from build123d import *

# Parameters (mm, degrees)
SKETCH_25_W          = 70
SKETCH_25_H          = 30
SKETCH_25_R          = 1.5
EXTRUDE_9_DEPTH      = 4
SKETCH_26_W          = 6
SKETCH_26_H          = 6
SKETCH_26_R          = 1.5
EXTRUDE_10_DEPTH     = 4
FILLET_3_R           = 1
EXTRUDE_11_DEPTH     = 6
SKETCH_28_W          = 6
SKETCH_28_H          = 18
EXTRUDE_12_DEPTH     = 2
SKETCH_29_R          = 5
CUT_EXTRUDE_15_DEPTH = 3
FILLET_4_R           = 5


with BuildPart() as part:
    # 草图25 → 凸台-拉伸9 (new body)
    with BuildSketch(Plane(origin=(0, 0, 0), x_dir=(1, 0, 0), z_dir=(0, 1, 0))):
        Rectangle(SKETCH_25_W, SKETCH_25_H)
        with Locations(Location((-32, 12, 0), (0, 0, 270))):
            Circle(SKETCH_25_R, mode=Mode.SUBTRACT)
        with Locations(Location((32, 12, 0), (0, 0, 270))):
            Circle(SKETCH_25_R, mode=Mode.SUBTRACT)
        with Locations(Location((32, -12, 0), (0, 0, 270))):
            Circle(SKETCH_25_R, mode=Mode.SUBTRACT)
        with Locations(Location((-32, -12, 0), (0, 0, 270))):
            Circle(SKETCH_25_R, mode=Mode.SUBTRACT)
    extrude(amount=EXTRUDE_9_DEPTH)

    # 草图26 → 凸台-拉伸10 (add)
    # profile 1 of 4: a face of its own
    with BuildSketch(Plane(origin=(0, 4, 0), x_dir=(1, 0, 0), z_dir=(0, 1, 0))):
        with Locations((-32, 12)):
            Rectangle(SKETCH_26_W, SKETCH_26_H)
        with Locations(Location((-32, 12, 0), (0, 0, 270))):
            Circle(SKETCH_26_R, mode=Mode.SUBTRACT)
    # profile 2 of 4: a face of its own
    with BuildSketch(Plane(origin=(0, 4, 0), x_dir=(1, 0, 0), z_dir=(0, 1, 0))):
        with Locations((-32, -12)):
            Rectangle(SKETCH_26_W, SKETCH_26_H)
        with Locations(Location((-32, -12, 0), (0, 0, 270))):
            Circle(SKETCH_26_R, mode=Mode.SUBTRACT)
    # profile 3 of 4: a face of its own
    with BuildSketch(Plane(origin=(0, 4, 0), x_dir=(1, 0, 0), z_dir=(0, 1, 0))):
        with Locations((32, -12)):
            Rectangle(SKETCH_26_W, SKETCH_26_H)
        with Locations(Location((32, -12, 0), (0, 0, 270))):
            Circle(SKETCH_26_R, mode=Mode.SUBTRACT)
    # profile 4 of 4: a face of its own
    with BuildSketch(Plane(origin=(0, 4, 0), x_dir=(1, 0, 0), z_dir=(0, 1, 0))):
        with Locations((32, 12)):
            Rectangle(SKETCH_26_W, SKETCH_26_H)
        with Locations(Location((32, 12, 0), (0, 0, 270))):
            Circle(SKETCH_26_R, mode=Mode.SUBTRACT)
    extrude(amount=EXTRUDE_10_DEPTH)

    # 圆角3
    fillet_3_edges = [part.edges().sort_by_distance(p)[0] for p in [
        (-35, 4, -15),
        (35, 4, -15),
        (35, 4, 15),
        (-35, 4, 15),
    ]]
    fillet(fillet_3_edges, radius=FILLET_3_R)

    # 草图27 → 凸台-拉伸11 (add)
    with BuildSketch(Plane.XZ):
        with BuildLine():
            Line((-42.4, 0), (-35, 0))
            Line((-35, 0), (-35, 10))
            Line((-35, 10), (-55, 10))
            Line((-55, 10), (-55, 0))
            Line((-55, 0), (-47.6, 0))
            ThreePointArc((-47.6, 0), (-45, 2.6), (-42.4, 0))
        make_face()
        with BuildLine():
            Line((-35, -10), (-35, 0))
            Line((-35, 0), (-42.4, 0))
            ThreePointArc((-42.4, 0), (-45, -2.6), (-47.6, 0))
            Line((-47.6, 0), (-55, 0))
            Line((-55, 0), (-55, -10))
            Line((-55, -10), (-35, -10))
        make_face()
        with BuildLine():
            ThreePointArc((42.4, 0), (45, 2.6), (47.6, 0))
            Line((47.6, 0), (55, 0))
            Line((55, 0), (55, 10))
            Line((55, 10), (35, 10))
            Line((35, 10), (35, 0))
            Line((35, 0), (42.4, 0))
        make_face()
        with BuildLine():
            Line((55, 0), (47.6, 0))
            ThreePointArc((47.6, 0), (45, -2.6), (42.4, 0))
            Line((42.4, 0), (35, 0))
            Line((35, 0), (35, -10))
            Line((35, -10), (55, -10))
            Line((55, -10), (55, 0))
        make_face()
    extrude(amount=-EXTRUDE_11_DEPTH)

    # 草图28 → 凸台-拉伸12 (add)
    with BuildSketch(Plane(origin=(0, 4, 0), x_dir=(1, 0, 0), z_dir=(0, 1, 0))):
        with Locations((-32, 0)):
            Rectangle(SKETCH_28_W, SKETCH_28_H)
        with Locations((32, 0)):
            Rectangle(SKETCH_28_W, SKETCH_28_H)
    extrude(amount=EXTRUDE_12_DEPTH)

    # 草图29 → 切除-拉伸15 (cut)
    with BuildSketch(Plane(origin=(0, 6, 0), x_dir=(1, 0, 0), z_dir=(0, 1, 0))):
        with Locations(Location((-45, 0, 0), (0, 0, 270))):
            Circle(SKETCH_29_R)
        with Locations(Location((45, 0, 0), (0, 0, 270))):
            Circle(SKETCH_29_R)
    extrude(amount=-CUT_EXTRUDE_15_DEPTH, mode=Mode.SUBTRACT)

    # 圆角4
    fillet_4_edges = [part.edges().sort_by_distance(p)[0] for p in [
        (-55, 3, -10),
        (-55, 3, 10),
        (55, 3, -10),
        (55, 3, 10),
    ]]
    fillet(fillet_4_edges, radius=FILLET_4_R)


solid = part.part
Verification items for the finished model (mm, model axes). A direction names the side the tool comes from. Coordinates: 2 decimals unless noted, no trailing zeros. Order: outer loops, then holes, each group sorted by start corner. A loop starts at its lowest first (then second) coordinate and runs counter-clockwise, first axis right, second up. Notation, with made-up numbers: M 44.25,86.5 L 71.25,86.5 A28 cw 71.25,118.5 Z; hole C 2.25,-11 d1. An arc over 180 degrees is marked long. Return JSON: item names as keys, results as strings.
1) Access from +Z, -Z, +X, -X, +Y, -Y to the whole of each face (thin tool, end or side, straight path). Record for faces 1 (the flat face through (-33.4, 8, 10.6)), 2 (the flat face through (32, 7, -9)).
Answer list:
{"face 1": "+Z, -Z, +X, -X, +Y", "face 2": "+X, -X, +Y"}
2) Thickness scan on L1, parallel to X at y = 4.75, z = 12; L2, parallel to X at y = 0.5, z = 12; L3, parallel to X at y = 4.2, z = 0. Record the ranges inside material, lowest first. Write a range as [from, to].
Answer list:
{"L1": "[-35, -33.5], [-30.5, -29], [29, 30.5], [33.5, 35]", "L2": "[-35, -33.5], [-30.5, 30.5], [33.5, 35]", "L3": "[-55, -50], [-40, -29], [29, 40], [50, 55]"}
3) Cross-section at A-A, the plane x = -32. Record the boundary of the cut face in (y, z), and give its area (3 significant figures).
Answer list:
{"outline": "M 0,-15 L 8,-15 L 8,-13.5 L 0,-13.5 Z; M 0,-10.5 L 8,-10.5 L 8,-9 L 6,-9 L 6,9 L 8,9 L 8,10.5 L 0,10.5 Z; M 0,13.5 L 8,13.5 L 8,15 L 0,15 Z", "area": "156 mm2"}
4) Cross-section at C-C, the plane y = 1. Record the boundary of the cut face in (x, z), and give its area (3 significant figures).
Answer list:
{"outline": "M -55,-5 A5 ccw -50,-10 L -35,-10 L -35,-14 A1 ccw -34,-15 L 34,-15 A1 ccw 35,-14 L 35,-10 L 50,-10 A5 ccw 55,-5 L 55,5 A5 ccw 50,10 L 35,10 L 35,14 A1 ccw 34,15 L -34,15 A1 ccw -35,14 L -35,10 L -50,10 A5 ccw -55,5 Z; hole C -45,0 d5.2; hole C -32,-12 d3; hole C -32,12 d3; hole C 32,-12 d3; hole C 32,12 d3; hole C 45,0 d5.2", "area": "2,810 mm2"}
5) Cross-section at D-D, the plane z = 12. Record the boundary of the cut face in (x, y), and give its area (3 significant figures).
Answer list:
{"outline": "M -35,0 L -33.5,0 L -33.5,8 L -35,8 Z; M -30.5,0 L 30.5,0 L 30.5,8 L 29,8 L 29,4 L -29,4 L -29,8 L -30.5,8 Z; M 33.5,0 L 35,0 L 35,8 L 33.5,8 Z", "area": "280 mm2"}
6) Cross-section at B-B, the plane x = 45. Record the boundary of the cut face in (y, z).
Answer list:
{"outline": "M 0,-10 L 6,-10 L 6,-5 L 3,-5 L 3,-2.6 L 0,-2.6 Z; M 0,2.6 L 3,2.6 L 3,5 L 6,5 L 6,10 L 0,10 Z"}
7) Release check for a two-part mould opening along Z. For faces 3 (the flat face through (-43, 3, -10)), 4 (the flat face through (-32, 7, 9)), 5 (the flat face through (30.6, 8, 10.6)), 6 (the flat face through (32, 7, 9)) record: +Z half, -Z half, draft (parallel to the pull), parting line (faces both ways), or undercut.
Answer list:
{"face 3": "-Z half", "face 4": "undercut", "face 5": "draft", "face 6": "undercut"}
8) Gauge pin test, flat ends, axial feed: pin 1 (3 mm diameter, centred on x = -37.5, y = 6, fed in from +Z); pin 2 (4 mm diameter, centred on y = 4, z = -10.5, fed in from +X); pin 3 (2 mm diameter, centred on x = 2, y = 6, fed in from -Z); pin 4 (5 mm diameter, centred on x = 32, z = -12, fed in from +Y). Record the tip position at first contact, or that the pin passes through.
Answer list:
{"pin 1": "z = 10", "pin 2": "x = 53.57", "pin 3": "through", "pin 4": "y = 8"}
